Part model, mm, in its own coordinate system. A direction names the side the tool comes from. Coordinates: 2 decimals unless noted, no trailing zeros. Loops run counter-clockwise (first coordinate to the right, second up) from the corner with the lowest first, then second, coordinate; pieces in that order, holes last. Notation, with made-up numbers: (30.25, 89.25) - (49.25, 89.25) arc R6 cw to (49.25, 95.25) - close; hole circle Ø10 at (72, 77). An arc over 180 degrees is marked (long way). Use a Markdown table: item, result. Add a question column.
1) Band-saw the part on A-A (x = -33.1). Give the cut face in (y, z).
2) Band-saw the part on D-D (x = 38.1). Give the cut face in (y, z), plus the area to 3 significant figures.
3) Pull direction Y, two halves, no side cores. Call faces 4 (the face through (6, -0.89, 29)), 5 (the face through (-36.1, -0.2, 10.5)), 6 (the face through (5.863, -22.157, 11.497)): +Y half, -Y half, draft (parallel to the pull), parting line (faces both ways), or undercut.
4) Drop flat-ended pins along their axis: P1, Ø4, axis at x = -22, y = -3.5, coming from the +Z side; P2, Ø3.5, axis at y = -5.5, z = 4.5, coming from the -X side; P3, Ø3.5, axis at x = -32.5, y = -17.5, coming from the -Z side. Give the stop position or say it passes through.
5) Probe probe 1 along Y at (x, z) = (-33, 23); probe 2 along X at (y, z) = (18.6, 23.25); probe 3 along Y at (x, z) = (35, 2.5). List the from-to ranges inside material, lowest first. Write a range as [from, to].
6) Tool access for faces 1 (the face through (34.73, 18.16, 8.11)), 2 (the face through (-31.99, -21.28, 21.93)), 3 (the face through (-22.866, -3.373, 9.943)): list every direction of +Z, -Z, +X, -X, +Y, -Y with a clear straight run to the whole face (end or side of a thin tool).
7) Band-saw the part on B-B (y = 18.6). Give the cut face in (x, z).
8) Band-saw the part on C-C (z = 26). Give the cut face in (x, y), plus the area to 3 significant figures.
Solid Edge part; units mm, degrees
sketch "Sketch1" plane through (0, 0, 0) normal (0, 0, 1) x (1, 0, 0)
  line L0 (-42.5, -23) -> (42.5, -23)
  line L1 (42.5, -23) -> (42.5, 23)
  line L2 (42.5, 23) -> (-42.5, 23)
  line L3 (-42.5, 23) -> (-42.5, -23)
  dimension "D1" = 42.5
  dimension "D2" = 42.5
extrude "Protrusion1" add sketch "Sketch1" along normal blind 27
sketch "Sketch2" plane through (0, 0, 27) normal (0, 0, 1) x (-1, 0, 0)
  line L0 (-33.11, 0.89) -> (21.89, 0.89)
  line L1 (21.89, 0.89) -> (21.89, -17.11)
  line L2 (21.89, -17.11) -> (-33.11, -17.11)
  line L3 (-33.11, -17.11) -> (-33.11, 0.89)
  dimension "D1" = 33.11
  dimension "D2" = 21.89
extrude "Extrusionsausprägung_2" add sketch "Sketch2" along normal blind 4
sketch "Sketch3" plane through (0, 0, 0) normal (0, 0, -1) x (1, 0, 0)
  line L0 (-5.89, 21.29) -> (-5.89, 23)
  line L1 (-7.39, 21.29) -> (-5.89, 21.29)
  line L2 (-7.39, 16.29) -> (-7.39, 21.29)
  line L3 (-14.39, 9.29) -> (-7.39, 16.29)
  line L4 (-14.39, -2.29) -> (-14.39, 9.29)
  line L5 (-22.89, -2.29) -> (-14.39, -2.29)
  line L6 (-22.89, -16.29) -> (-22.89, -2.29)
  line L7 (-7.39, -16.29) -> (-22.89, -16.29)
  line L8 (-7.39, -21.29) -> (-7.39, -16.29)
  line L9 (-5.89, -21.29) -> (-7.39, -21.29)
  line L10 (-5.89, -23) -> (-5.89, -21.29)
  line L11 (5.61, -23) -> (-5.89, -23)
  dimension "D1" = 5.89
  dimension "D2" = 7.39
  dimension "D3" = 5.89
  dimension "D4" = 7.39
  dimension "D5" = 22.89
revolve "RevolvedCutout1" cut sketch "Sketch3" angle 360 about axis through (5.61, 23, 0) along (0, -1, 0) material side at (-5.84, -22.145, 0)
sketch "Sketch4" plane through (-24.195, 0, 0) normal (0, 0, -1) x (0, -1, 0)
  line L0 (0, 5.355) -> (12, 5.355)
  line L1 (12, 5.355) -> (12, 0.255)
  line L2 (12, 0.255) -> (0, 0.255)
  dimension "D1" = 12
revolve "RevolvedCutout2" cut sketch "Sketch4" angle 360 about axis through (-42.5, 0, 0) along (1, 0, 0)
sketch "Sketch5" plane through (-24.195, 0, 0) normal (0, 0, -1) x (1, 0, 0)
  line L0 (-0.255, 0) -> (-0.255, 10.5)
  line L1 (-0.255, 10.5) -> (3.745, 10.5)
  line L2 (3.745, 10.5) -> (16.745, 7.5)
  line L3 (16.745, 7.5) -> (16.745, 0)
  line L4 (16.745, 0) -> (-0.255, 0)
  dimension "D1" = 0.255
revolve "RevolvedCutout3" cut sketch "Sketch5" angle 360 about axis through (-42.5, 0, 0) along (1, 0, 0)
sketch "Sketch6" plane through (-24.195, 0, 0) normal (0, 0, -1) x (1, 0, 0)
  line L0 (-18.305, 0) -> (-5.355, 0)
  line L1 (-5.355, 0) -> (-5.355, -10.5)
  line L2 (-5.355, -10.5) -> (-18.305, -10.5)
  line L3 (-18.305, -10.5) -> (-18.305, 0)
revolve "RevolvedCutout4" cut sketch "Sketch6" angle 360 about axis through (0, 0, 0) along (1, 0, 0)
hole "Bohrung_9" at (38.1, 18.6, 27) direction (0, 0, -1) diameter 5.8 depth 10
hole "Hole1" at (38.1, -18.6, 27) direction (0, 0, -1) diameter 5.8 depth 10
hole "Hole2" at (-33.1, -18.6, 27) direction (0, 0, -1) diameter 5.8 depth 10
hole "Hole3" at (-33.1, 18.6, 27) direction (0, 0, -1) diameter 5.8 depth 10
hole "Bohrung_1" at (38.1, -18.6, 0) direction (0, 0, 1) diameter 6.8 depth 16
hole "Hole4" at (38.1, 18.6, 0) direction (0, 0, 1) diameter 6.8 depth 16
hole "Hole5" at (-33.1, 18.6, 0) direction (0, 0, 1) diameter 6.8 depth 16
hole "Hole6" at (-33.1, -18.6, 0) direction (0, 0, 1) diameter 6.8 depth 16
properties material "Polykarbonat"
Answer block:
| question | item | result |
|---|---|---|
| 1 | outline | (-23, 0) - (-22, 0) - (-22, 16) - (-15.2, 16) - (-15.2, 0) - (-10.5, 0) arc R10.5 cw to (10.5, 0) - (15.2, 0) - (15.2, 16) - (22, 16) - (22, 0) - (23, 0) - (23, 27) - (21.5, 27) - (21.5, 17) - (15.7, 17) - (15.7, 27) - (-15.7, 27) - (-15.7, 17) - (-21.5, 17) - (-21.5, 27) - (-23, 27) - close |
| 2 | outline | (-23, 0) - (-22, 0) - (-22, 16) - (-15.2, 16) - (-15.2, 0) - (15.2, 0) - (15.2, 16) - (22, 16) - (22, 0) - (23, 0) - (23, 27) - (21.5, 27) - (21.5, 17) - (15.7, 17) - (15.7, 27) - (-15.7, 27) - (-15.7, 17) - (-21.5, 17) - (-21.5, 27) - (-23, 27) - close |
| 2 | area | 908 mm2 |
| 3 | face 4 | -Y half |
| 3 | face 5 | undercut |
| 3 | face 6 | draft |
| 4 | P1 | z = 27 |
| 4 | P2 | x = 24.61 |
| 4 | P3 | z = 16 |
| 5 | probe 1 | [-23, -21.5], [-15.7, 15.7], [21.5, 23] |
| 5 | probe 2 | [-42.5, -36], [-30.2, 35.2], [41, 42.5] |
| 5 | probe 3 | [-23, -20], [-17.2, 17.2], [20, 23] |
| 6 | face 1 | -Z |
| 6 | face 2 | +Z |
| 6 | face 3 | -Z, -X |
| 7 | outline | (-42.5, 0) - (-36.5, 0) - (-36.5, 16) - (-29.7, 16) - (-29.7, 0) - (-7.39, 0) arc R13 cw to (18.61, 0) - (34.7, 0) - (34.7, 16) - (41.5, 16) - (41.5, 0) - (42.5, 0) - (42.5, 27) - (41, 27) - (41, 17) - (35.2, 17) - (35.2, 27) - (-30.2, 27) - (-30.2, 17) - (-36, 17) - (-36, 27) - (-42.5, 27) - close |
| 8 | outline | (-42.5, -23) - (42.5, -23) - (42.5, 23) - (-42.5, 23) - close; hole circle Ø5.8 at (-33.1, -18.6); hole circle Ø5.8 at (-33.1, 18.6); hole (-6.06, 2.29) - (17.28, 2.29) - (17.28, 16.29) - (-6.06, 16.29) - close; hole circle Ø5.8 at (38.1, -18.6); hole circle Ø5.8 at (38.1, 18.6) |
| 8 | area | 3,480 mm2 |
